Here's how the part is built. I have some questions about the finished solid (model axes, mm). Round coordinates to 2 decimals unless told otherwise and drop trailing zeros. Write each loop counter-clockwise with the first axis right and the second up, starting at its lowest first coordinate (ties: lowest second). Pieces come first, ordered by that corner, then holes. Notation, with made-up numbers: M 50,59 L 77,59 A21 cw 77,92 Z; hole C 56.5,-26.5 d8. An arc over 180 degrees is marked long. Use one line per item in the form item = value. Start each with the question number.
Q1. I want a section at A-A on z = 0. List the corners of the cut face in (x, y) for me, and give its area (3 significant figures).
Q2. I need wall thicknesses on line 1 along X through (y, z) = (2.75, 0); line 2 along Z through (x, y) = (0, 1.7); line 3 along Z through (x, y) = (0.75, 3.2). Which ranges of each line are inside material? Lowest first, please. Write a range as from..to.
Q3. I want a section at B-B on x = 0. List the corners of the cut face in (y, z) for me, and give its area (3 significant figures).
Q4. We'd pull the mould along X, two halves only. Please class faces 1 (the face through (0, 0, -6)), 2 (the face through (0.191, 2.021, -4.496)), 3 (the face through (0.202, 1.979, -4.746)): +X half, -X half, draft (parallel to the pull), parting line (faces both ways), or undercut.
Q5. I want a section at D-D on y = 2.85. List the corners of the cut face in (x, z) for me.
Q6. I'm going to push flat-ended pins straight in: pin 1 Ø3.5 at (x, z) = (-3, 1.5) entering from -Y; pin 2 Ø1 at (y, z) = (1.5, -2) entering from +X; pin 3 Ø1.5 at (y, z) = (1.5, -2) entering from +X. Where does each tip first touch, or does it pass through?
Q7. I want a section at C-C on x = 3.5. List the corners of the cut face in (y, z) for me.
```python
from build123d import *

# Parameters (mm, degrees)
CUT_EXTRUDE_1_DEPTH = 0.5
CUT_EXTRUDE_2_DEPTH = 4.5
FILLET_1_R          = 0.25
FILLET_2_R          = 0.5


with BuildPart() as part:
    # Эскиз1 → Повернуть1 (revolve)
    with BuildSketch(Plane.XY):
        Polygon((4.5, 0), (4.5, 3.5), (4.75, 3.5), (4.75, 0.25), (7.75, 0.25), (7.75, 0), align=None)
    revolve(axis=Axis((0, 0, 0), (0, 1, 0)))

    # Эскиз2 → Вырез-Вытянуть1 (cut)
    with BuildSketch(Plane.XZ):
        with BuildLine():
            Line((-1.5, -7.603453163), (-1.5, -2.4))
            Line((-1.5, -2.4), (1.5, -2.4))
            Line((1.5, -2.4), (1.5, -7.603453163))
            ThreePointArc((1.5, -7.603453163), (0, 7.75), (-1.5, -7.603453163))
        make_face()
    extrude(amount=-CUT_EXTRUDE_1_DEPTH, mode=Mode.SUBTRACT)

    # Эскиз3 → Вырез-Вытянуть2 (cut, through all)
    with BuildSketch(Plane(origin=(0, 3.5, 0), x_dir=(1, 0, 0), z_dir=(0, 1, 0))):
        with BuildLine():
            ThreePointArc((0.5, -4.472135955), (0, -4.5), (-0.5, -4.472135955))
            Line((-0.5, -4.472135955), (-0.5, -4.723610907))
            ThreePointArc((-0.5, -4.723610907), (0, -4.75), (0.5, -4.723610907))
            Line((0.5, -4.723610907), (0.5, -4.472135955))
        make_face()
    extrude(amount=-CUT_EXTRUDE_2_DEPTH, mode=Mode.SUBTRACT)

    # Скругление1
    fillet_1_edges = [part.edges().sort_by_distance(p)[0] for p in [
        (0, 0.25, -4.75),
    ]]
    fillet(fillet_1_edges, radius=FILLET_1_R)

    # Скругление2
    fillet_2_edges = [part.edges().sort_by_distance(p)[0] for p in [
        (0, 0, -4.5),
    ]]
    fillet(fillet_2_edges, radius=FILLET_2_R)


solid = part.part
```
Reported:
q1.outline = M -4.75,0.5 L -4.5,0.5 L -4.5,3.5 L -4.75,3.5 Z; M 4.5,0.5 L 4.75,0.5 L 4.75,3.5 L 4.5,3.5 Z
q1.area = 1.50 mm^2
q2.line_1 = -4.75..-4.5, 4.5..4.75
q2.line_2 = -4.75..-4.5
q2.line_3 = -4.69..-4.44, 4.44..4.69
q3.outline = M 0,-7.75 L 0.25,-7.75 L 0.25,-5 A0.25 cw 0.5,-4.75 L 3.5,-4.75 L 3.5,-4.5 L 0.5,-4.5 A0.5 ccw 0,-5 Z
q3.area = 1.58 mm^2
q4.face_1 = draft
q4.face_2 = undercut
q4.face_3 = parting line
q5.outline = M -0.5,4.47 L -0.5,4.72 A4.75 ccw long 0.5,4.72 L 0.5,4.47 A4.5 cw long Z
q6.pin_1 = 0.5
q6.pin_2 = 4.51
q6.pin_3 = 4.58
q7.outline = M 0.5,-3.21 L 3.5,-3.21 L 3.5,-2.83 L 0.5,-2.83 Z; M 0.5,2.83 L 3.5,2.83 L 3.5,3.21 L 0.5,3.21 Z
